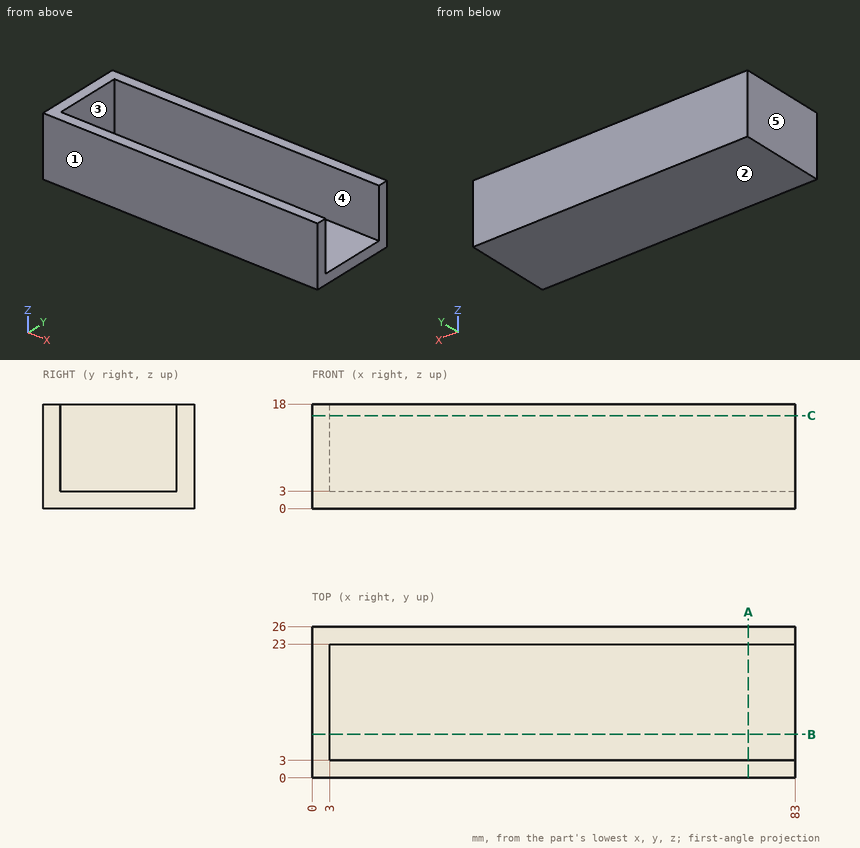
Part print with two shaded views. Sizes in mm from the minimum x, y, z corner. A direction names the side the tool comes from. Round coordinates to 2 decimals unless told otherwise and drop trailing zeros. Order: outer loops, then holes, each group sorted by start corner. A loop starts at its lowest first (then second) coordinate and runs counter-clockwise, first axis right, second up.
(1) Pull direction Y, two halves, no side cores. Call the marked faces 1, 2 and 3: released by +Y, released by -Y, zero draft, split by the parting line, or undercut.
(2) Band-saw the part on C-C (z = 16). List the corners of the cut face in (x, y), then the cut area to 3 significant figures.
(3) Band-saw the part on A-A (x = 75). List the corners of the cut face in (y, z), then the cut area to 3 significant figures.
(4) Pin check, flat tips, straight feed: pin 1 (1.5 mm diameter, centred on x = 31, y = 11.5, fed in from +Z); pin 2 (3 mm diameter, centred on y = 8.5, z = 12.5, fed in from +X). Stop position of each tip, or through.
(5) Drill centre lines: line 1 (Y direction, x = 45.5, z = 4); line 2 (Z direction, x = 18, y = 19). Where is each one in solid material? Low to high.
(6) 3-axis set-ups, long thin cutter, end or side, ignore diameter. For the marked faces 4 and 5: which of +Z, -Z, +X, -X, +Y, -Y reach the whole face in a straight line?
(7) Band-saw the part on B-B (y = 7.5). List the corners of the cut face in (x, z).
Verdict:
1. face 1: released by -Y
1. face 2: zero draft
1. face 3: undercut
2. outline: (0, 0) - (83, 0) - (83, 3) - (3, 3) - (3, 23) - (83, 23) - (83, 26) - (0, 26) - close
2. area: 558 mm2
3. outline: (0, 0) - (26, 0) - (26, 18) - (23, 18) - (23, 3) - (3, 3) - (3, 18) - (0, 18) - close
3. area: 168 mm2
4. pin 1: stops at z = 3
4. pin 2: stops at x = 3
5. line 1: y = 0 to 3, 23 to 26
5. line 2: z = 0 to 3
6. face 4: +Z, +X
6. face 5: +Z, -Z, -X, +Y, -Y
7. outline: (0, 0) - (83, 0) - (83, 3) - (3, 3) - (3, 18) - (0, 18) - close
